Geometry: final body of the model. Coordinates: model frame, mm. Give positions to 0.01 mm unless a question says otherwise; leave off trailing zeros. Order: outer loops, then holes, each group sorted by start corner. A loop starts at its lowest first (then second) coordinate and runs counter-clockwise, first axis right, second up. Notation, with made-up numbers: (73.25, 83) -> (132.25, 83) arc R22 ccw to (132.25, 109) -> close; hole circle Ø7 at (-28, 35.5). An arc over 180 degrees is marked (long way). One line per item, written item: value. Start each with the question number.
```python
from build123d import *

# Parameters (mm, degrees)
SKETCH1_W                 = 12.7
SKETCH1_H                 = 6.0198
BOSS_EXTRUDE1_DEPTH       = 6.35
SKETCH13_R                = 0.635
CUT_EXTRUDE2_DEPTH        = 6.35
CHAMFER1_SIZE             = 50.8
FILLET2_R                 = 12.7
F_4_CLEARANCE_HOLE1_D     = 2.9464
F_4_CLEARANCE_HOLE1_DEPTH = 6.35
F_4_CLEARANCE_HOLE1_TIP   = 0.885187864
CUT_EXTRUDE3_REACH        = 164.372
SKETCH14_R                = 1.9685
F_4_CLEARANCE_HOLE2_D     = 2.9464
F_4_CLEARANCE_HOLE2_DEPTH = 6.35
F_4_CLEARANCE_HOLE2_TIP   = 0.885187864
CUT_EXTRUDE4_REACH        = 164.372
F_4_CLEARANCE_HOLE3_D     = 2.9464
F_4_CLEARANCE_HOLE3_DEPTH = 6.35
F_4_CLEARANCE_HOLE3_TIP   = 0.885187864


with BuildPart() as part:
    # Sketch1 → Boss-Extrude1 (new body)
    with BuildSketch(Plane.XY):
        Polygon((-25.4, 0), (25.4, 0), (25.4, -6.35), (38.1, -6.35), (38.1, 0), (44.45, 0), (44.45, 77.052), (88.9, 77.052), (88.9, 80.227), (101.6, 80.227), (101.6, 77.052), (114.3, 77.052), (114.3, 115.152), (101.6, 115.152), (101.6, 111.977), (88.9, 111.977), (88.9, 115.152), (-44.45, 115.152), (-44.45, 0), (-38.1, 0), (-38.1, -6.35), (-25.4, -6.35), align=None)
        with Locations((12.7, 9.3599)):
            Rectangle(SKETCH1_W, SKETCH1_H, mode=Mode.SUBTRACT)
        with Locations((-12.7, 9.3599)):
            Rectangle(SKETCH1_W, SKETCH1_H, mode=Mode.SUBTRACT)
    extrude(amount=BOSS_EXTRUDE1_DEPTH)

    # Sketch13 → Cut-Extrude2 (cut)
    with BuildSketch(Plane.XY):
        with Locations((-19.05, 12.3698)):
            Circle(SKETCH13_R)
    cut_extrude2 = extrude(amount=CUT_EXTRUDE2_DEPTH, mode=Mode.SUBTRACT)

    # Sketch-Pattern1: Cut-Extrude2 at 11 more places
    with Locations((12.7, 0, 0), (12.7, -6.0198, 0), (0, -6.0198, 0), (25.4, 0, 0), (38.1, 0, 0), (38.1, -6.0198, 0), (25.4, -6.0198, 0), (57.15, -12.3698, 0), (44.45, -12.3698, 0), (-6.35, -12.3698, 0), (-19.05, -12.3698, 0)):
        add(cut_extrude2, mode=Mode.SUBTRACT)

    # Chamfer1
    chamfer1_edges = [part.edges().sort_by_distance(p)[0] for p in [
        (-44.45, 115.152, 3.175),
    ]]
    chamfer(chamfer1_edges, length=CHAMFER1_SIZE)

    # Fillet2
    fillet2_edges = [part.edges().sort_by_distance(p)[0] for p in [
        (44.45, 77.052, 3.175),
    ]]
    fillet(fillet2_edges, radius=FILLET2_R)

    # #4 Clearance Hole1
    with Locations(Plane.XY.offset(6.35)):
        with Locations((-31.75, 3.175), (31.75, 3.175), (0, 3.175)):
            Hole(F_4_CLEARANCE_HOLE1_D / 2, depth=F_4_CLEARANCE_HOLE1_DEPTH)
            with Locations((0, 0, -(F_4_CLEARANCE_HOLE1_DEPTH + F_4_CLEARANCE_HOLE1_TIP / 2))):  # 118° drill point
                Cone(0, F_4_CLEARANCE_HOLE1_D / 2, F_4_CLEARANCE_HOLE1_TIP, mode=Mode.SUBTRACT)

    # Sketch14 → Cut-Extrude3 (cut, up to next)
    with BuildSketch(Plane.XY.offset(6.35), mode=Mode.PRIVATE) as cut_extrude3_sk1:
        with Locations((95.25, 86.577)):
            Circle(SKETCH14_R)
    cut_extrude3_tool1 = extrude(cut_extrude3_sk1.sketch, amount=-CUT_EXTRUDE3_REACH, mode=Mode.PRIVATE) & part.part
    # Sketch14 → Cut-Extrude3 (cut, up to next)
    with BuildSketch(Plane.XY.offset(6.35), mode=Mode.PRIVATE) as cut_extrude3_sk2:
        with Locations((82.55, 80.227)):
            Circle(SKETCH14_R)
    cut_extrude3_tool2 = extrude(cut_extrude3_sk2.sketch, amount=-CUT_EXTRUDE3_REACH, mode=Mode.PRIVATE) & part.part
    # Sketch14 → Cut-Extrude3 (cut, up to next)
    with BuildSketch(Plane.XY.offset(6.35), mode=Mode.PRIVATE) as cut_extrude3_sk3:
        with Locations((107.95, 80.227)):
            Circle(SKETCH14_R)
    cut_extrude3_tool3 = extrude(cut_extrude3_sk3.sketch, amount=-CUT_EXTRUDE3_REACH, mode=Mode.PRIVATE) & part.part
    add(cut_extrude3_tool1.solids().sort_by_distance((95.25, 86.577, 6.35))[0], mode=Mode.SUBTRACT)
    add(cut_extrude3_tool2.solids().sort_by_distance((82.55, 80.227, 6.35))[0], mode=Mode.SUBTRACT)
    add(cut_extrude3_tool3.solids().sort_by_distance((107.95, 80.227, 6.35))[0], mode=Mode.SUBTRACT)

    # #4 Clearance Hole2
    with Locations(Plane.XY.offset(6.35)):
        with Locations((63.5, 83.402), (63.5, 108.802)):
            Hole(F_4_CLEARANCE_HOLE2_D / 2, depth=F_4_CLEARANCE_HOLE2_DEPTH)
            with Locations((0, 0, -(F_4_CLEARANCE_HOLE2_DEPTH + F_4_CLEARANCE_HOLE2_TIP / 2))):  # 118° drill point
                Cone(0, F_4_CLEARANCE_HOLE2_D / 2, F_4_CLEARANCE_HOLE2_TIP, mode=Mode.SUBTRACT)

    # Sketch18 → Cut-Extrude4 (cut, up to next)
    with BuildSketch(Plane.XY.offset(6.35), mode=Mode.PRIVATE) as cut_extrude4_sk1:
        with BuildLine():
            Line((6.35, 96.8375), (31.75, 96.8375))
            ThreePointArc((31.75, 96.8375), (39.6875, 88.9), (31.75, 80.9625))
            Line((31.75, 80.9625), (6.35, 80.9625))
            ThreePointArc((6.35, 80.9625), (-1.5875, 88.9), (6.35, 96.8375))
        make_face()
    cut_extrude4_tool1 = extrude(cut_extrude4_sk1.sketch, amount=-CUT_EXTRUDE4_REACH, mode=Mode.PRIVATE) & part.part
    add(cut_extrude4_tool1.solids().sort_by_distance((19.05, 88.9, 6.35))[0], mode=Mode.SUBTRACT)

    # #4 Clearance Hole3
    with Locations(Plane.XY.offset(6.35)):
        with Locations((-4.7625, 88.9), (42.8625, 88.9)):
            Hole(F_4_CLEARANCE_HOLE3_D / 2, depth=F_4_CLEARANCE_HOLE3_DEPTH)
            with Locations((0, 0, -(F_4_CLEARANCE_HOLE3_DEPTH + F_4_CLEARANCE_HOLE3_TIP / 2))):  # 118° drill point
                Cone(0, F_4_CLEARANCE_HOLE3_D / 2, F_4_CLEARANCE_HOLE3_TIP, mode=Mode.SUBTRACT)


solid = part.part
```
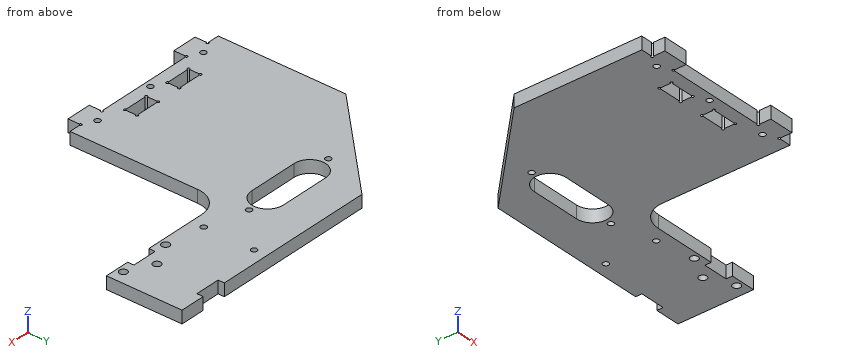
1. Cut plane B-B, the plane y = 43.5. Return loops of the section in (x, z).
2. Cut plane C-C, the plane z = 1. State how many separate pieces and enclosed holes the cut face has, then the cut area to 3 significant figures.
3. Cut plane D-D, the plane x = 48.5. Return loops of the section in (y, z).
4. Cut plane A-A, the plane x = 107.95. Return loops of the section in (y, z), then the cut area to 3 significant figures.
5. Material intervals for L1, parallel to Y at x = 63.5, z = 4; L2, parallel to X at y = 3, z = 1.5; L3, parallel to X at y = 11.5, z = 1.25, sorted ascending. Write a range as [from, to].
6. Pin query (flat end, axial travel): P1, Ø0.8, axis at x = -38.1, y = 0, coming from the +Z side; P2, Ø1.9, axis at x = 107.5, z = 3.5, coming from the -Y side. Return the tip coordinate at first contact, or that it passes through.
Answers follow:
1. outline: (-44.45, 0) -> (44.45, 0) -> (44.45, 6.35) -> (-44.45, 6.35) -> close
2. separate pieces: 1
2. enclosed holes: 13
2. area: 10,900 mm²
3. outline: (73.65, 0) -> (115.15, 0) -> (115.15, 6.35) -> (73.65, 6.35) -> close
4. outline: (77.05, 0) -> (78.26, 0) -> (78.26, 6.35) -> (77.05, 6.35) -> close; (82.2, 0) -> (115.15, 0) -> (115.15, 6.35) -> (82.2, 6.35) -> close
4. area: 217 mm²
5. L1: y = [77.05, 81.93], [84.88, 107.33], [110.28, 115.15]
5. L2: x = [-44.45, -33.21], [-30.29, -1.46], [1.46, 30.29], [33.21, 44.45]
5. L3: x = [-44.45, -19.05], [-6.35, 6.35], [19.05, 44.45]
6. P1: passes through
6. P2: stops at y = 77.05
